Geometry: final body of the model. Coordinates: model frame, mm. Round coordinates to 2 decimals unless told otherwise and drop trailing zeros. Order: outer loops, then holes, each group sorted by start corner. A loop starts at its lowest first (then second) coordinate and runs counter-clockwise, first axis right, second up. Notation, with made-up numbers: (-9, 73.5) - (-4, 73.5) arc R6 cw to (-4, 79.5) - close; hole circle Ø10 at (-21.75, -1). An arc over 180 degrees is marked (long way). Put each result on its own line as item: value. Start each with the question number.
(1) Section A-A (y = 0). Output: boundary loops of the cut face in (x, z), and give its area (3 significant figures).
(2) Section D-D (x = 7). Output: boundary loops of the cut face in (y, z), and give its area (3 significant figures).
(3) Material intervals for L1, parallel to Z at x = 7.5, y = 8; L2, parallel to Z at x = 3, y = -16; L3, parallel to Y at x = 11.25, z = 0.5, sorted ascending. Write a range as [from, to].
(4) Pin query (flat end, axial travel): P1, Ø3, axis at x = 2.5, y = -2.5, coming from the -Z side; P2, Ø3, axis at x = 2, z = -7, coming from the +Y side; P3, Ø2, axis at x = 4, y = -3.5, coming from the -Z side. Return the tip coordinate at first contact, or that it passes through.
(5) Section C-C (x = 10). Output: boundary loops of the cut face in (y, z), and give its area (3 significant figures).
(6) Pull-direction query (Y, two-part tool) for faces 1 (the face through (5.875, -4.769, 21.477)), 2 (the face through (0, -5, -18)), 3 (the face through (1.073, -3.869, -17.424)); classes: released by +Y, released by -Y, zero draft, split by the parting line, or undercut.
Solid Edge part; units mm, degrees
sketch "Sketch1" plane through (0, 0, 0) normal (0, 0, 1) x (1, 0, 0)
  arc A0 (0, 17.9546) -> (0.3768, 17.6646) centre (0.3, 17.9546) ccw
  line L0 (0.3768, 17.6646) -> (11.5, 20.6103)
  line L1 (11.5, 20.6103) -> (11.5, 21.8)
  arc A1 (11.5, 21.8) -> (11.3, 22) centre (11.3, 21.8) ccw
  line L2 (11.3, 22) -> (0.6, 22)
  arc A2 (0.6, 22) -> (0, 21.4) centre (0.6, 21.4) ccw
  line L3 (0, 21.4) -> (0, 17.9546)
revolve "RevolvedProtrusion1" add sketch "Sketch1" angle 360 about axis through (11.5, 0, 0) along (-1, 0, 0)
properties part number "320/22 X_or"
Checks:
1. outline: (0, -21.4) arc R0.6 ccw to (0.6, -22) - (11.3, -22) arc R0.2 ccw to (11.5, -21.8) - (11.5, -20.61) - (0.38, -17.66) arc R0.3 ccw to (0, -17.95) - close; (0, 17.95) arc R0.3 ccw to (0.38, 17.66) - (11.5, 20.61) - (11.5, 21.8) arc R0.2 ccw to (11.3, 22) - (0.6, 22) arc R0.6 ccw to (0, 21.4) - close
1. area: 66.7 mm²
2. outline: circle Ø44 at (0, 0); hole circle Ø38.84 at (0, 0)
2. area: 336 mm²
3. L1: z = [-20.49, -17.84], [17.84, 20.49]
3. L2: z = [-15.1, -9], [9, 15.1]
3. L3: y = [-21.99, -20.54], [20.54, 21.99]
4. P1: stops at z = -21.98
4. P2: stops at y = 21.3
4. P3: stops at z = -21.86
5. outline: circle Ø44 at (0, 0); hole circle Ø40.43 at (0, 0)
5. area: 237 mm²
6. face 1: split by the parting line
6. face 2: zero draft
6. face 3: undercut
